For this review, take the finished solid that the model builds, in its own axes (mm). Face numbers are marked on the shaded views. A direction names the side the tool comes from. Give positions to 0.01 mm unless a question says otherwise; leave off trailing zeros. Write each loop counter-clockwise with the first axis right and the second up, starting at its lowest first coordinate (ties: lowest second). Pieces come first, ordered by that corner, then holes. Notation, with made-up numbers: (14.5, 70) -> (47.5, 70) arc R23 ccw to (47.5, 90) -> close; hole circle Ø10 at (-32, 28). An arc over 180 degrees is marked (long way). Answer as CSV lines item,"result".
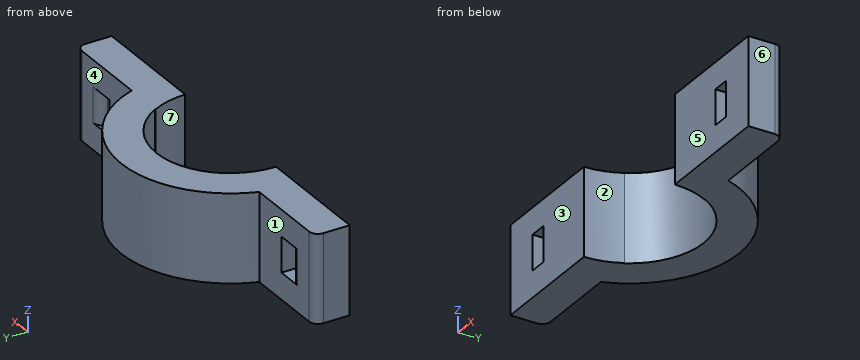
```python
from build123d import *

# Parameters (mm, degrees)
BOSS_EXTRUDE1_DEPTH = 12.7
SKETCH3_W           = 12.7
SKETCH3_H           = 5.08
BOSS_EXTRUDE2_DEPTH = 27.94
SKETCH4_R           = 10.668
CUT_EXTRUDE1_DEPTH  = 44.196
CUT_EXTRUDE3_REACH  = 36.524
SKETCH6_W           = 2.54
SKETCH6_H           = 5.08
FILLET1_R           = 1.27


with BuildPart() as part:
    # Sketch2 → Boss-Extrude1 (new body)
    with BuildSketch(Plane.XY):
        with BuildLine():
            Line((-15.8115, 0), (-10.7315, 0))
            ThreePointArc((-10.7315, 0), (0, 10.7315), (10.7315, 0))
            Line((10.7315, 0), (15.8115, 0))
            ThreePointArc((15.8115, 0), (0, 15.8115), (-15.8115, 0))
        make_face()
    extrude(amount=BOSS_EXTRUDE1_DEPTH)

    # Sketch3 → Boss-Extrude2 (add, symmetric)
    with BuildSketch(Plane(origin=(0, 0, 0), x_dir=(0, 0, -1), z_dir=(1, 0, 0))):
        with Locations((-6.35, 2.54)):
            Rectangle(SKETCH3_W, SKETCH3_H)
    extrude(amount=BOSS_EXTRUDE2_DEPTH, both=True)

    # Sketch4 → Cut-Extrude1 (cut)
    with BuildSketch(Plane.XY.offset(12.7)):
        Circle(SKETCH4_R)
    extrude(amount=-CUT_EXTRUDE1_DEPTH, mode=Mode.SUBTRACT)

    # Sketch6 → Cut-Extrude3 (cut, up to next)
    with BuildSketch(Plane.XZ, mode=Mode.PRIVATE) as cut_extrude3_sk1:
        with Locations((-21.456606913, 6.35)):
            Rectangle(SKETCH6_W, SKETCH6_H)
    cut_extrude3_tool1 = extrude(cut_extrude3_sk1.sketch, amount=-CUT_EXTRUDE3_REACH, mode=Mode.PRIVATE) & part.part
    # Sketch6 → Cut-Extrude3 (cut, up to next)
    with BuildSketch(Plane.XZ, mode=Mode.PRIVATE) as cut_extrude3_sk2:
        with Locations((21.456606913, 6.35)):
            Rectangle(SKETCH6_W, SKETCH6_H)
    cut_extrude3_tool2 = extrude(cut_extrude3_sk2.sketch, amount=-CUT_EXTRUDE3_REACH, mode=Mode.PRIVATE) & part.part
    add(cut_extrude3_tool1.solids().sort_by_distance((-21.456607, 0, 6.35))[0], mode=Mode.SUBTRACT)
    add(cut_extrude3_tool2.solids().sort_by_distance((21.456607, 0, 6.35))[0], mode=Mode.SUBTRACT)

    # Fillet1
    fillet1_edges = [part.edges().sort_by_distance(p)[0] for p in [
        (-27.94, 5.08, 6.35),
        (27.94, 5.08, 6.35),
        (-22.726606913, 5.08, 6.35),
        (22.726606913, 5.08, 6.35),
    ]]
    fillet(fillet1_edges, radius=FILLET1_R)


solid = part.part
```
Q1. Clearance check with flat-ended pins moving along their axes: pin 1 (4 mm diameter, centred on y = 10, z = 10.5, fed in from -X); pin 2 (2 mm diameter, centred on y = 6.5, z = 7.5, fed in from +X); pin 3 (2 mm diameter, centred on y = 4, z = 2, fed in from -X); pin 4 (6 mm diameter, centred on x = 21, z = 3.5, fed in from +Y). State where each tip first meets the part, or that it passes through.
Answer block:
pin 1,"stops at x = -13.64"
pin 2,"stops at x = 14.82"
pin 3,"stops at x = -27.94"
pin 4,"stops at y = 5.08"
Q2. For the marked faces 1, 2, 3 and 4, list the 3-axis set-ups (+Z, -Z, +X, -X, +Y, -Y) from which the entire face can be reached by the end or side of a thin tool; tool diameter is ignored.
Answer block:
face 1,"+Z, -Z, -X, +Y"
face 2,"+Z, -Z, -Y"
face 3,"+Z, -Z, +X, -X, -Y"
face 4,"+Z, -Z, +X, +Y"
Q3. To check wall thickness, follow probe 1 along Z at (x, y) = (21, 3.25); probe 2 along X at (y, z) = (4.75, 5.75); probe 3 along Y at (x, z) = (-16.5, 4.75). State the ranges of each line that lie inside material, in increasing order. Write a range as [from, to].
Answer block:
probe 1,"z = [0, 3.81], [8.89, 12.7]"
probe 2,"x = [-27.52, -23.14], [-20.19, -9.55], [9.55, 20.19], [23.14, 27.52]"
probe 3,"y = [0, 5.08]"
Q4. Draft analysis for pull direction X (two halves, no side actions). For the marked faces 5, 6 and 7, state which applies: released by +X, released by -X, zero draft, split by the parting line, or undercut.
Answer block:
face 5,"zero draft"
face 6,"released by +X"
face 7,"undercut"
Q5. Add section C-C (y = 9.25). Write out the cut boundary in (x, z).
Answer block:
outline,"(-12.82, 0) -> (-5.44, 0) -> (-5.44, 12.7) -> (-12.82, 12.7) -> close; (5.44, 0) -> (12.82, 0) -> (12.82, 12.7) -> (5.44, 12.7) -> close"
Q6. Add section D-D (z = 11.75). Write out the cut boundary in (x, y).
Answer block:
outline,"(-27.94, 0) -> (-10.67, 0) arc R10.67 cw to (-9.38, 5.08) -> (-9.45, 5.08) arc R10.73 cw to (9.45, 5.08) -> (9.38, 5.08) arc R10.67 cw to (10.67, 0) -> (27.94, 0) -> (27.94, 3.81) arc R1.27 ccw to (26.67, 5.08) -> (14.97, 5.08) arc R15.81 ccw to (-14.97, 5.08) -> (-26.67, 5.08) arc R1.27 ccw to (-27.94, 3.81) -> close"
Q7. Add section B-B (y = 1.5). Write out the cut boundary in (x, z), plus the area to 3 significant figures.
Answer block:
outline,"(-27.94, 0) -> (-10.56, 0) -> (-10.56, 12.7) -> (-27.94, 12.7) -> close; (10.56, 0) -> (27.94, 0) -> (27.94, 12.7) -> (10.56, 12.7) -> close; hole (-22.73, 3.81) -> (-20.19, 3.81) -> (-20.19, 8.89) -> (-22.73, 8.89) -> close; hole (20.19, 3.81) -> (22.73, 3.81) -> (22.73, 8.89) -> (20.19, 8.89) -> close"
area,"416 mm2"
Q8. Add section A-A (z = 5.25). Write out the cut boundary in (x, y).
Answer block:
outline,"(-27.94, 0) -> (-22.73, 0) -> (-22.73, 3.81) arc R1.27 ccw to (-24, 5.08) -> (-26.67, 5.08) arc R1.27 ccw to (-27.94, 3.81) -> close; (-20.19, 0) -> (-10.67, 0) arc R10.67 cw to (-9.38, 5.08) -> (-9.45, 5.08) arc R10.73 cw to (9.45, 5.08) -> (9.38, 5.08) arc R10.67 cw to (10.67, 0) -> (20.19, 0) -> (20.19, 5.08) -> (14.97, 5.08) arc R15.81 ccw to (-14.97, 5.08) -> (-20.19, 5.08) -> close; (22.73, 0) -> (27.94, 0) -> (27.94, 3.81) arc R1.27 ccw to (26.67, 5.08) -> (24, 5.08) arc R1.27 ccw to (22.73, 3.81) -> close"
